from build123d import *

# Parameters (mm, degrees)
SKETCH001_R        = 1.5
POCKET_DEPTH       = 156.780455
POCKET_DEPTH_BACK  = 128.780455
POLARPATTERN_COUNT = 4


with BuildPart() as part:
    # Sketch → Revolution (revolve)
    with BuildSketch(Plane.XZ):
        Polygon((5, -25), (5, -14), (4.25, -14), (4.25, 14), (5, 14), (5, 25), (11, 25), (11, 10), (5.5, 10), (5.5, -10), (11, -10), (11, -25), align=None)
    revolve(axis=Axis((0, 0, 0), (0, 0, 1)))

    # Sketch001 (on Face2 of Revolution) → Pocket (cut, two sides)
    with BuildSketch(Plane(origin=(0, 0, -14), x_dir=(1, 0, 0), z_dir=(0, 0, -1))) as pocket_sk:
        with Locations((0, 8)):
            Circle(SKETCH001_R)
    pocket = extrude(amount=-POCKET_DEPTH, mode=Mode.SUBTRACT) + extrude(pocket_sk.sketch, amount=POCKET_DEPTH_BACK, mode=Mode.SUBTRACT)

    # PolarPattern: Pocket ×4 about axis
    polarpattern_axis = Axis((0, 0, -14), (0, 0, -1))
    for i in range(1, POLARPATTERN_COUNT):
        add(pocket.rotate(polarpattern_axis, i * 360 / POLARPATTERN_COUNT), mode=Mode.SUBTRACT)


solid = part.part
The listing builds one solid part. Answer for the finished solid, in the listing's coordinates (mm). A direction names the side the tool comes from. Coordinates: 2 decimals unless noted, no trailing zeros. Order: outer loops, then holes, each group sorted by start corner. A loop starts at its lowest first (then second) coordinate and runs counter-clockwise, first axis right, second up. Notation, with made-up numbers: M 86,-32.5 L 109,-32.5 A16 ccw 109,-5.5 Z; hole C 45,55 d2. An arc over 180 degrees is marked long. Use CSV: the item, a comma, the result in double quotes.
Q1. Straight lines are drawn through the part: L1, parallel to Y at x = 0, z = 22.25; L2, parallel to Z at x = 5, y = -6.75; L3, parallel to Y at x = -3.25, z = 21.5. For each, find the intervals that lie inside material, in ascending order.
Here are the results:
L1,"-11 to -9.5, -6.5 to -5, 5 to 6.5, 9.5 to 11"
L2,"-25 to -10, 10 to 25"
L3,"-10.51 to -3.8, 3.8 to 10.51"
Q2. Section D-D (y = 3.5) is taken. Determine the outline of the cut face in (x, z).
Here are the results:
outline,"M -10.43,-25 L -3.57,-25 L -3.57,-14 L -2.41,-14 L -2.41,14 L -3.57,14 L -3.57,25 L -10.43,25 L -10.43,10 L -4.24,10 L -4.24,-10 L -10.43,-10 Z; M 2.41,-14 L 3.57,-14 L 3.57,-25 L 10.43,-25 L 10.43,-10 L 4.24,-10 L 4.24,10 L 10.43,10 L 10.43,25 L 3.57,25 L 3.57,14 L 2.41,14 Z"
Q3. Section C-C (z = -17) is taken. Determine the outline of the cut face in (x, y), then the cut area to 3 significant figures.
Here are the results:
outline,"C 0,0 d22; hole C -8,0 d3; hole C 0,0 d10; hole C 0,-8 d3; hole C 0,8 d3; hole C 8,0 d3"
area,"273 mm2"
Q4. Given pin 1 Ø2.5 at (x, y) = (0, 8) entering from -Z; pin 2 Ø6 at (y, z) = (-8, 8.5) entering from -X; pin 3 Ø1 at (x, y) = (-3, 3) entering from +Z; pin 4 Ø4 at (y, z) = (4, -14) entering from -X, each flat-ended and moving along its own axis, determine where each tip first touches the part or whether it passes through.
Here are the results:
pin 1,"through"
pin 2,"x = -9.58"
pin 3,"z = 14"
pin 4,"x = -10.82"
Q5. Determine the mould class of faces 1 (the cylindrical face through (-1.19, -5.37, -0.14)), 2 (the flat face through (-3, 5, 10)), 3 (the cylindrical face through (-1.08, -4.88, 19.58)) for opening direction Y: pulls with the +Y half, pulls with the -Y half, needs draft (parallel to the pull), parting line crosses it, or undercut.
Here are the results:
face 1,"parting line crosses it"
face 2,"needs draft"
face 3,"undercut"
Q6. Section A-A (x = -8) is taken. Determine the outline of the cut face in (y, z).
Here are the results:
outline,"M -7.55,-25 L -1.5,-25 L -1.5,-10 L -7.55,-10 Z; M -7.55,10 L -1.5,10 L -1.5,25 L -7.55,25 Z; M 1.5,-25 L 7.55,-25 L 7.55,-10 L 1.5,-10 Z; M 1.5,10 L 7.55,10 L 7.55,25 L 1.5,25 Z"
Q7. A tool of negligible diameter and unlimited length cuts with its end or side. For faces 4 (the cylindrical face through (-2.38, -10.74, -17.6)), 5 (the flat face through (-2, -4, -14)), 6 (the flat face through (3, 5, -10)), from which of +Z, -Z, +X, -X, +Y, -Y can it reach the whole face along a straight path? Write none if from no direction.
Here are the results:
face 4,"+Z, -Z"
face 5,"-Z"
face 6,"none"
